from build123d import *

# Parameters (mm, degrees)
BOSS_EXTRUDE1_DEPTH = 9
SKETCH2_R           = 1
CUT_EXTRUDE1_DEPTH  = 36.693136595
SKETCH3_R           = 1.5
CUT_EXTRUDE2_DEPTH  = 26.889186932


with BuildPart() as part:
    # Sketch1 → Boss-Extrude1 (new body)
    with BuildSketch(Plane(origin=(0, 0, 0), x_dir=(1, 0, 0), z_dir=(0, 1, 0))):
        Polygon((-20.5, 13), (-9.5, 13), (-9.5, 0), (9.5, 0), (9.5, 13), (20.5, 13), (20.5, 11), (11.5, 11), (11.5, -2), (-11.5, -2), (-11.5, 11), (-20.5, 11), align=None)
    extrude(amount=BOSS_EXTRUDE1_DEPTH)

    # Sketch2 → Cut-Extrude1 (cut, through all)
    with BuildSketch(Plane.ZY.offset(11.5)):
        with Locations((-9, 4.5)):
            Circle(SKETCH2_R)
    extrude(amount=-CUT_EXTRUDE1_DEPTH, mode=Mode.SUBTRACT)

    # Sketch3 → Cut-Extrude2 (cut, through all)
    with BuildSketch(Plane.XY.offset(-11)):
        with Locations((-16, 4.5)):
            Circle(SKETCH3_R)
        with BuildLine():
            Line((-20.5, 9), (-20.5, 4.5))
            ThreePointArc((-20.5, 4.5), (-19.181980515, 7.681980515), (-16, 9))
            Line((-16, 9), (-20.5, 9))
        make_face()
        with BuildLine():
            Line((20.5, 4.5), (20.5, 9))
            Line((20.5, 9), (16, 9))
            ThreePointArc((16, 9), (19.181980515, 7.681980515), (20.5, 4.5))
        make_face()
        with Locations((16, 4.5)):
            Circle(SKETCH3_R)
    extrude(amount=-CUT_EXTRUDE2_DEPTH, mode=Mode.SUBTRACT)


solid = part.part
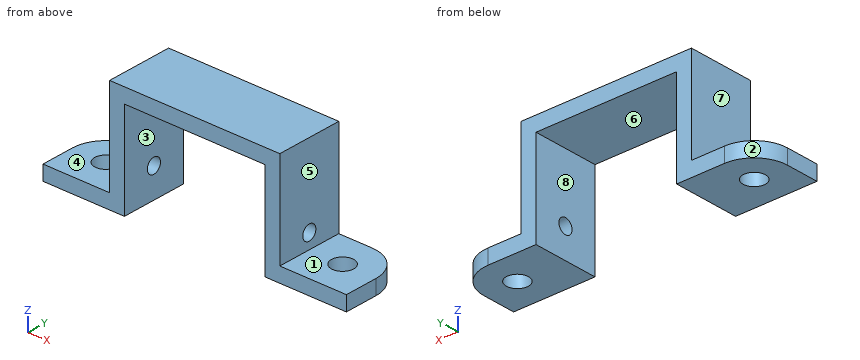
Work out the finished part from the listing and answer in its coordinate system (mm). Face numbers are marked on the shaded views. A direction names the side the tool comes from. Round coordinates to 2 decimals unless told otherwise and drop trailing zeros. Write each loop counter-clockwise with the first axis right and the second up, starting at its lowest first coordinate (ties: lowest second). Pieces come first, ordered by that corner, then holes. Notation, with made-up numbers: (46, -6) -> (58, -6) arc R22 ccw to (58, 9) -> close; hole circle Ø9 at (7, -34.5). An arc over 180 degrees is marked (long way). Write each question's results on one line, items separated by ' | '.
Item 1: Flat-ended cylindrical pins translate along their axes: P1, Ø4.5, axis at y = 5.5, z = -6, coming from the -X side; P2, Ø5, axis at x = 10.5, z = -4, coming from the -Y side; P3, Ø2.5, axis at x = 14.5, y = 3.5, coming from the +Z side. Find the tip coordinate at first contact, or state that the pin passes through.
Result set:
P1: x = -11.5 | P2: y = 0 | P3: z = -11
Item 2: A cutting plane is placed at D-D, the plane y = 7.75. Determine the outline of the cut face in (x, z).
Result set:
outline: (-19.11, -13) -> (-9.5, -13) -> (-9.5, 0) -> (9.5, 0) -> (9.5, -13) -> (19.11, -13) -> (19.11, -11) -> (11.5, -11) -> (11.5, 2) -> (-11.5, 2) -> (-11.5, -11) -> (-19.11, -11) -> close
Item 3: A cutting plane is placed at C-C, the plane y = 4. Determine the outline of the cut face in (x, z), plus the area to 3 significant figures.
Result set:
outline: (-20.5, -13) -> (-17.41, -13) -> (-17.41, -11) -> (-20.5, -11) -> close; (-14.59, -13) -> (-9.5, -13) -> (-9.5, -9.87) -> (-11.5, -9.87) -> (-11.5, -11) -> (-14.59, -11) -> close; (-11.5, -8.13) -> (-9.5, -8.13) -> (-9.5, 0) -> (9.5, 0) -> (9.5, -8.13) -> (11.5, -8.13) -> (11.5, 2) -> (-11.5, 2) -> close; (9.5, -13) -> (14.59, -13) -> (14.59, -11) -> (11.5, -11) -> (11.5, -9.87) -> (9.5, -9.87) -> close; (17.41, -13) -> (20.5, -13) -> (20.5, -11) -> (17.41, -11) -> close | area: 116 mm^2
Item 4: Which of the six approach directions +Z, -Z, +X, -X, +Y, -Y give full straight-line access (tool end or side, diameter ignored) to the marked faces 1, 2, 3 and 4?
Result set:
face 1: +Z, +X, +Y, -Y | face 2: +Z, -Z, -X, +Y | face 3: -Z, +Y, -Y | face 4: +Z, -X, +Y, -Y
Item 5: A cutting plane is placed at B-B, the plane z = -9. Determine the outline of the cut face in (x, y), plus the area to 3 significant figures.
Result set:
outline: (-11.5, 0) -> (-9.5, 0) -> (-9.5, 3.5) -> (-11.5, 3.5) -> close; (-11.5, 5.5) -> (-9.5, 5.5) -> (-9.5, 9) -> (-11.5, 9) -> close; (9.5, 0) -> (11.5, 0) -> (11.5, 3.5) -> (9.5, 3.5) -> close; (9.5, 5.5) -> (11.5, 5.5) -> (11.5, 9) -> (9.5, 9) -> close | area: 28.0 mm^2
Item 6: Find the intervals of material crossed by line 1 along Y through (x, z) = (-10.65, -9); line 2 along X through (y, z) = (7.75, -4.5); line 3 along Y through (x, z) = (-16, -12.25), in increasing order. Write a range as [from, to].
Result set:
line 1: [0, 3.5], [5.5, 9] | line 2: [-11.5, -9.5], [9.5, 11.5] | line 3: [0, 3], [6, 9]
Item 7: A cutting plane is placed at A-A, the plane z = -4.5. Determine the outline of the cut face in (x, y), plus the area to 3 significant figures.
Result set:
outline: (-11.5, 0) -> (-9.5, 0) -> (-9.5, 9) -> (-11.5, 9) -> close; (9.5, 0) -> (11.5, 0) -> (11.5, 9) -> (9.5, 9) -> close | area: 36.0 mm^2
Item 8: The mould has two halves that part along X. Classify the marked faces 5, 6, 7 and 8: +X half, -X half, draft (parallel to the pull), parting line (faces both ways), or undercut.
Result set:
face 5: +X half | face 6: undercut | face 7: -X half | face 8: undercut
